Autodesk Inventor part; units mm, degrees
ref_plane "工作平面5" through (7.5, 0, 0) normal (1, 0, 0) x (0, 1, 0)
ref_plane "XZ Plane" through (0, 0, 0) normal (0, 1, 0) x (-1, 0, 0)
ref_plane "XY Plane" through (0, 0, 0) normal (0, 0, 1) x (1, 0, 0)
sketch "草圖1" plane through (0, 0, 0) normal (0, 0, 1) x (1, 0, 0)
  line L0 (0, 0) -> (80, 0)
  line L1 (80, 0) -> (80, 150)
  line L2 (0, 110) -> (0, 0)
  line L3 (80, 150) -> (0, 110)
  line L4 (0, 70) -> (80, 70)
  dimension "d3" = 70
  dimension "d4" = 40
  dimension "d5" = 80
  dimension "d73" = 80
extrude "擠出1" add sketch "草圖1" along normal mid plane 80
sketch "草圖5" plane through (0, 0, 40) normal (-1, 0, 0) x (0, 0, 1)
  circle A0 centre (-40, 40) radius 15
  line L0 (-80, 0) -> (0, 0)
  line L1 (-40, -30) -> (-40, 180)
  point P0 (-40, 0)
  dimension "d24" = 40
  dimension "d25" = 30
extrude "擠出5" cut sketch "草圖5" against normal through all
sketch "草圖11" plane through (0, 0, 0) normal (1, 0, 0) x (0, 1, 0)
  line L0 (150, -40) -> (150, 40)
  line L1 (80, -20) -> (150, -20)
  line L2 (150, -20) -> (150, 20)
  line L3 (150, 20) -> (80, 20)
  line L4 (80, 20) -> (80, -20)
  line L5 (80, -20) -> (150, 20) construction
  line L6 (150, -20) -> (80, 20) construction
  line L7 (-28, 0) -> (168, 0)
  line L8 (0, -40) -> (0, 40)
  point P0 (0, 0)
  point P1 (115, 0)
  point P2 (115, 0)
  dimension "d55" = 40
  dimension "d56" = 80
extrude "擠出11" cut sketch "草圖11" along normal through all
ref_plane "工作平面5" through (7.5, 0, 0) normal (1, 0, 0) x (0, 1, 0)
sketch "草圖12" plane through (7.5, 0, 0) normal (1, 0, 0) x (0, 1, 0)
  line L0 (0, -40) -> (0, 40)
  line L1 (80, -30) -> (0, -30)
  line L2 (0, -30) -> (0, 30)
  line L3 (0, 30) -> (80, 30)
  line L4 (80, 30) -> (80, -30)
  circle A0 centre (40, 0) radius 15
  line L5 (80, -30) -> (0, 30) construction
  line L6 (0, -30) -> (80, 30) construction
  point P0 (0, 0)
  dimension "d60" = 60
extrude "擠出12" cut sketch "草圖12" along normal blind 65
sketch "草圖13" plane through (7.5, 0, 0) normal (1, 0, 0) x (0, 1, 0)
  line L0 (150, -40) -> (150, -20)
  line L1 (150, -20) -> (80, -20)
  line L2 (80, -20) -> (80, -25)
  line L3 (80, -25) -> (150, -25)
  line L4 (150, -25) -> (150, -20)
  line L5 (0, 0) -> (140, 0) construction
  line L6 (150, 40) -> (150, 20)
  line L7 (150, 20) -> (80, 20)
  line L8 (80, 25) -> (150, 25)
  line L9 (150, 25) -> (150, 20)
  line L10 (80, 20) -> (80, -20)
  line L11 (80, -20) -> (80, 20)
  line L12 (80, 20) -> (80, 25)
  dimension "d72" = 5
extrude "擠出13" cut sketch "草圖13" along normal blind 5
pattern_linear "矩形陣列3" count 4 spacing 20 along (1, 0, 0) of "擠出13"
properties part number "架"
Source: CAD feature listing. Evaluate the final solid. Frame: model axes, mm. A direction names the side the tool comes from. Round coordinates to 2 decimals unless told otherwise and drop trailing zeros. Loops run counter-clockwise (first coordinate to the right, second up) from the corner with the lowest first, then second, coordinate; pieces in that order, holes last.
(1) Section query D-D (z = -18). Output: boundary loops of the cut face in (x, y).
From the geometry:
outline: (0, 0) - (7.5, 0) - (7.5, 80) - (0, 80) - close; (72.5, 0) - (80, 0) - (80, 80) - (72.5, 80) - close
(2) Contact query for a flat-ended pin moving along its axis: pin 1 Ø2 at (x, z) = (71, -25) entering from -Y. Output: stop coordinate, or through.
From the geometry:
pin 1: stops at y = 80
(3) Material intervals for probe 1 along Y at (x, z) = (74, 0); probe 2 along Z at (x, y) = (66, 134); probe 3 along X at (y, z) = (135, 24.5), sorted ascending.
From the geometry:
probe 1: y = 0 to 25, 55 to 80
probe 2: z = -40 to -20, 20 to 40
probe 3: x = 52.5 to 67.5, 72.5 to 80
(4) Pull-direction query (X, two-part tool) for faces 1 (the flat face through (80, 57, -1)), 2 (the flat face through (4, 97, -20)), 3 (the flat face through (47.5, 106, 23)); classes: +X half, -X half, draft (parallel to the pull), parting line (faces both ways), or undercut.
From the geometry:
face 1: +X half
face 2: draft
face 3: undercut
(5) Section query A-A (z = 0). Output: boundary loops of the cut face in (x, y), and give its area (3 significant figures).
From the geometry:
outline: (0, 0) - (7.5, 0) - (7.5, 25) - (0, 25) - close; (0, 55) - (7.5, 55) - (7.5, 80) - (0, 80) - close; (72.5, 0) - (80, 0) - (80, 25) - (72.5, 25) - close; (72.5, 55) - (80, 55) - (80, 80) - (72.5, 80) - close
area: 750 mm2
(6) Section query C-C (y = 140). Output: boundary loops of the cut face in (x, z), and give its area (3 significant figures).
From the geometry:
outline: (60, -40) - (80, -40) - (80, -20) - (72.5, -20) - (72.5, -25) - (67.5, -25) - (67.5, -20) - (60, -20) - close; (60, 20) - (67.5, 20) - (67.5, 25) - (72.5, 25) - (72.5, 20) - (80, 20) - (80, 40) - (60, 40) - close
area: 750 mm2
(7) Section query B-B (x = 57.5). Output: boundary loops of the cut face in (y, z).
From the geometry:
outline: (0, -40) - (138.75, -40) - (138.75, -20) - (80, -20) - (80, -30) - (0, -30) - close; (0, 30) - (80, 30) - (80, 20) - (138.75, 20) - (138.75, 40) - (0, 40) - close
(8) Access query for faces 4 (the flat face through (76, 115, -20)), 5 (the flat face through (7.5, 31, 14)), 6 (the flat face through (70, 113, 25)), 7 (the flat face through (40.6, 130.3, 29.9)). Directions: +Z, -Z, +X, -X, +Y, -Y. A direction counts if a zero-diameter tool reaches every point of the face in a straight line with its end or side. Return the directions, or none.
From the geometry:
face 4: +X, -X, +Y
face 5: -Y
face 6: +Y, -Y
face 7: +Z, -Z, -X, +Y
